Here's the drawing with two shaded views (mm, measured from the low corner). I have some questions. Round coordinates to 2 decimals unless told otherwise and drop trailing zeros. Write each loop counter-clockwise with the first axis right and the second up, starting at its lowest first coordinate (ties: lowest second). Pieces come first, ordered by that corner, then holes. Notation, with made-up numbers: M 16.5,83 L 66.5,83 A22 ccw 66.5,111 Z; hole C 74,45.25 d11. An arc over 180 degrees is marked long. Answer as a JSON object with one key per item and string values. Group by question number.
1) Suppose I cut it at C-C, the plane z = 6. Write out the boundary of the cut face in (x, y) (1 decimal).
2) If we mould it in two halves opening along X, with no side actions, what happens to the marked faces 1, 2 and 3? For each: +X half, -X half, draft (parallel to the pull), parting line (faces both ways), or undercut.
3) Suppose I cut it at A-A, the plane y = 3.75. Write out the boundary of the cut face in (x, z) (1 decimal).
4) Please list where these lines run through material, in increasing order: L1, parallel to Y at x = 3.5, z = 14.75 (1 decimal); L2, parallel to Y at x = 4.5, z = 12.75 (1 decimal). Write a range as [from, to].
5) Suppose I cut it at D-D, the plane x = 6.25. Write out the boundary of the cut face in (y, z) (1 decimal).
6) I'm going to push a flat-ended pin straight in: pin 1 Ø1 at (y, z) = (6, 11.5) entering from -X. Where does the tip first touch, or does it pass through?
7) Suppose I cut it at B-B, the plane x = 4. Write out the boundary of the cut face in (y, z) (1 decimal).
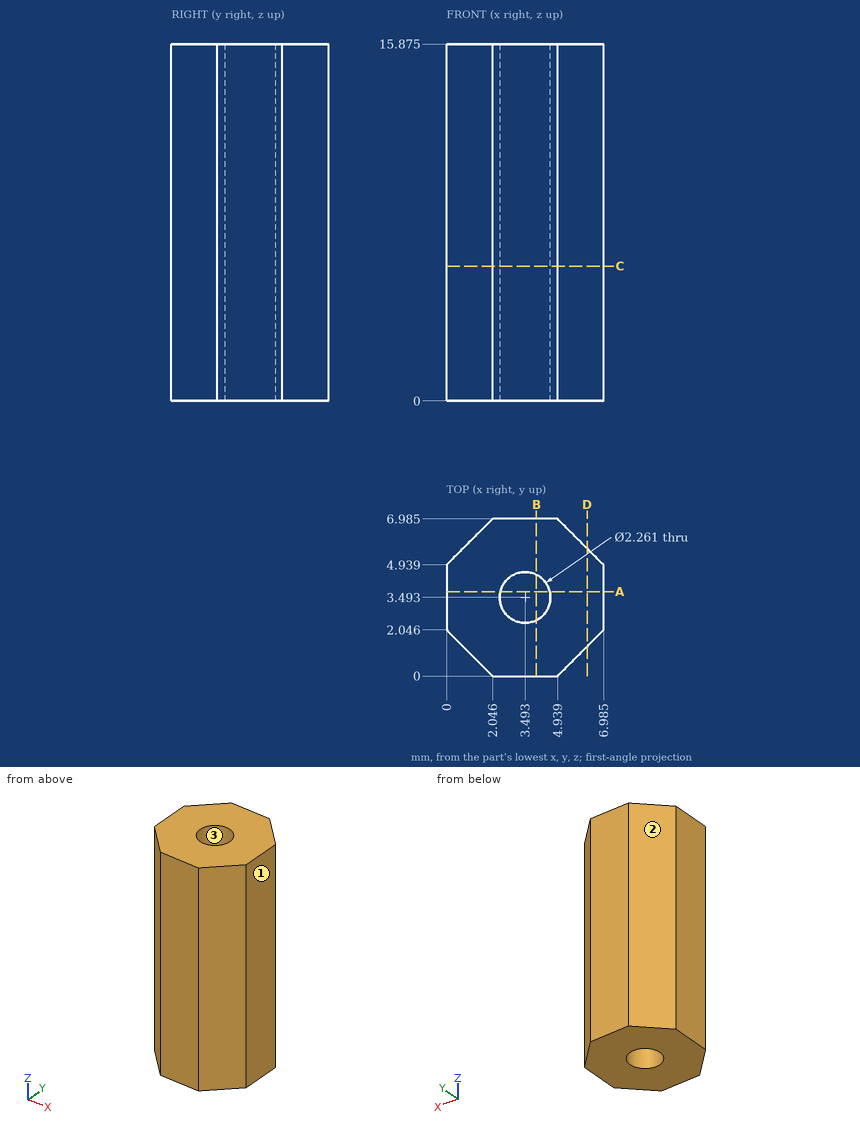
Results:
{
 "1": {"outline": "M 0,2 L 2,0 L 4.9,0 L 7,2 L 7,4.9 L 4.9,7 L 2,7 L 0,4.9 Z; hole C 3.5,3.5 d2.3"},
 "2": {"face 1": "+X half", "face 2": "-X half", "face 3": "undercut"},
 "3": {"outline": "M 0,0 L 2.4,0 L 2.4,15.9 L 0,15.9 Z; M 4.6,0 L 7,0 L 7,15.9 L 4.6,15.9 Z"},
 "4": {"L1": "[0, 2.4], [4.6, 7]", "L2": "[0, 3], [4, 7]"},
 "5": {"outline": "M 1.3,0 L 5.7,0 L 5.7,15.9 L 1.3,15.9 Z"},
 "6": {"pin 1": "x = 0.56"},
 "7": {"outline": "M 0,0 L 2.5,0 L 2.5,15.9 L 0,15.9 Z; M 4.5,0 L 7,0 L 7,15.9 L 4.5,15.9 Z"}
}
